```python
from build123d import *

# Parameters (mm, degrees)
F0_W     = 19.05
F0_H     = 3.175
F1_DEPTH = 9.525
F2_W     = 50.8
F2_H     = 6.35
F3_DEPTH = 12.7
F5_DEPTH = 273.051
F7_DEPTH = 19.05
F8_DEPTH = 19.05


with BuildPart() as f1:
    # F0 (on Top) → F1 (new body, symmetric)
    with BuildSketch(Plane.XY):
        Polygon((-127, 0), (127, 0), (127, 9.525), (-127, 9.525), (-127, 3.175), align=None)
        Polygon((-127, -3.175), (-127, -9.525), (127, -9.525), (127, 0), (-127, 0), align=None)
        with Locations((-136.525, 1.5875)):
            Rectangle(F0_W, F0_H)
        with Locations((-136.525, -1.5875)):
            Rectangle(F0_W, F0_H)
    extrude(amount=F1_DEPTH, both=True)

    # F2 (on Top) → F3 (cut, symmetric)
    with BuildSketch(Plane.XY):
        with Locations((101.6, 6.35)):
            Rectangle(F2_W, F2_H)
        with Locations((101.6, -6.35)):
            Rectangle(F2_W, F2_H)
    extrude(amount=F3_DEPTH, both=True, mode=Mode.SUBTRACT)

    # F4 (on face) → F5 (cut, through all)
    with BuildSketch(Plane.YZ.offset(127)):
        with BuildLine():
            ThreePointArc((-9.525, 0), (-7.77713, 5.499261), (-3.175, 8.980256))
            Line((-3.175, 8.980256), (-3.175, 9.525))
            Line((-3.175, 9.525), (-9.525, 9.525))
            Line((-9.525, 9.525), (-9.525, 0))
        make_face()
        with BuildLine():
            Line((-3.175, -9.525), (-3.175, -8.980256))
            ThreePointArc((-3.175, -8.980256), (-7.77713, -5.499261), (-9.525, 0))
            Line((-9.525, 0), (-9.525, -9.525))
            Line((-9.525, -9.525), (-3.175, -9.525))
        make_face()
        with BuildLine():
            Line((9.525, -9.525), (9.525, 0))
            ThreePointArc((9.525, 0), (7.77713, -5.499261), (3.175, -8.980256))
            Line((3.175, -8.980256), (3.175, -9.525))
            Line((3.175, -9.525), (9.525, -9.525))
        make_face()
        with BuildLine():
            ThreePointArc((3.175, 8.980256), (7.77713, 5.499261), (9.525, 0))
            Line((9.525, 0), (9.525, 9.525))
            Line((9.525, 9.525), (3.175, 9.525))
            Line((3.175, 9.525), (3.175, 8.980256))
        make_face()
        with BuildLine():
            ThreePointArc((0, 9.525), (1.610696, 9.387826), (3.175, 8.980256))
            Line((3.175, 8.980256), (3.175, 9.525))
            Line((3.175, 9.525), (0, 9.525))
        make_face()
        with BuildLine():
            ThreePointArc((-3.175, 8.980256), (-1.610696, 9.387826), (0, 9.525))
            Line((0, 9.525), (-3.175, 9.525))
            Line((-3.175, 9.525), (-3.175, 8.980256))
        make_face()
        with BuildLine():
            Line((-3.175, -9.525), (0, -9.525))
            ThreePointArc((0, -9.525), (-1.610696, -9.387826), (-3.175, -8.980256))
            Line((-3.175, -8.980256), (-3.175, -9.525))
        make_face()
        with BuildLine():
            Line((3.175, -9.525), (3.175, -8.980256))
            ThreePointArc((3.175, -8.980256), (1.610696, -9.387826), (0, -9.525))
            Line((0, -9.525), (3.175, -9.525))
        make_face()
    extrude(amount=-F5_DEPTH, mode=Mode.SUBTRACT)

    # F6 (on face) → F7 (cut)
    with BuildSketch(Plane(origin=(-146.05, 0, 0), x_dir=(0, -1, 0), z_dir=(-1, 0, 0))):
        with BuildLine():
            ThreePointArc((-3.175, 0), (0, 3.175), (3.175, 0))
            Line((3.175, 0), (3.175, 8.980256))
            ThreePointArc((3.175, 8.980256), (1.610696, 9.387826), (0, 9.525))
            ThreePointArc((0, 9.525), (-1.610696, 9.387826), (-3.175, 8.980256))
            Line((-3.175, 8.980256), (-3.175, 0))
        make_face()
    extrude(amount=-F7_DEPTH, mode=Mode.SUBTRACT)

    # F6 (on face) → F8 (cut)
    with BuildSketch(Plane(origin=(-146.05, 0, 0), x_dir=(0, -1, 0), z_dir=(-1, 0, 0))):
        with BuildLine():
            Line((3.175, -8.980256), (3.175, 0))
            ThreePointArc((3.175, 0), (0, -3.175), (-3.175, 0))
            Line((-3.175, 0), (-3.175, -8.980256))
            ThreePointArc((-3.175, -8.980256), (-1.610696, -9.387826), (0, -9.525))
            ThreePointArc((0, -9.525), (1.610696, -9.387826), (3.175, -8.980256))
        make_face()
    extrude(amount=-F8_DEPTH, mode=Mode.SUBTRACT)


solid = f1.part
```
Read the model definition and answer for the solid it produces. Units are mm, in the model's axes. A direction names the side the tool comes from. Coordinates: 2 decimals unless noted, no trailing zeros. Order: outer loops, then holes, each group sorted by start corner. A loop starts at its lowest first (then second) coordinate and runs counter-clockwise, first axis right, second up. Notation, with made-up numbers: (-30.75, -30.5) - (-19.75, -30.5) arc R14 ccw to (-19.75, -26.5) - close; hole circle Ø11 at (-34.75, 31). An arc over 180 degrees is marked (long way). Answer as a JSON object with one key per item and string values. Group by question number.
Item 1: Section C-C (y = 5.75) is taken. Give the vertices of the cut face in (x, z), plus the area to 3 significant figures.
Item 2: Section A-A (x = -44) is taken. Give the vertices of the cut face in (y, z) (3 decimals), plus the area to 3 significant figures.
Item 3: Section D-D (y = -7.25) is taken. Give the vertices of the cut face in (x, z), plus the area to 3 significant figures.
Item 4: A tool of negligible diameter and unlimited length cuts with its end or side. For faces 1 (the face through (76.2, 6, 0)), 2 (the face through (76.2, -6, 0)), 3 (the face through (-127, -4, 0)), 4 (the face through (-146.05, 0, 0)), 5 (the face through (127, 0, 0)), from which of +Z, -Z, +X, -X, +Y, -Y can it reach the whole face along a straight path? Write none if from no direction.
Item 5: Flat-ended cylindrical pins translate along their axes: P1, Ø1.5, axis at x = -1, y = -1, coming from the +Z side; P2, Ø1, axis at y = 7.5, z = -0.5, coming from the -X side; P3, Ø3, axis at y = 5, z = -2, coming from the +X side; P4, Ø5, axis at x = -39, z = 2.5, coming from the +Y side (3 decimals). Find the tip coordinate at first contact, or state that the pin passes through.
Item 6: Section B-B (z = -6.25) is taken. Give the vertices of the cut face in (x, y) (3 decimals), plus the area to 3 significant figures.
Item 7: Consider probe 1 along X at (y, z) = (-1, 4.5); probe 2 along X at (y, z) = (3.75, -1.75); probe 3 along Y at (x, z) = (116.5, 6) (3 decimals). Determine where each line is inside the solid, lowest interval first. Write a range as from..to.
Results are:
{
 "1": {"outline": "(-127, -7.59) - (76.2, -7.59) - (76.2, 7.59) - (-127, 7.59) - close", "area": "3,090 mm^2"},
 "2": {"outline": "(-3.175, -8.98) arc R9.525 ccw to (0, -9.525) arc R9.525 ccw to (3.175, -8.98) arc R9.525 ccw to (3.175, 8.98) arc R9.525 ccw to (0, 9.525) arc R9.525 ccw to (-3.175, 8.98) arc R9.525 ccw to start", "area": "285 mm^2"},
 "3": {"outline": "(-127, -6.18) - (76.2, -6.18) - (76.2, 6.18) - (-127, 6.18) - close", "area": "2,510 mm^2"},
 "4": {"face 1": "+Z, -Z, +X, +Y", "face 2": "+Z, -Z, +X, -Y", "face 3": "-X", "face 4": "+Z, -Z, -X, +Y, -Y", "face 5": "+Z, -Z, +X, +Y, -Y"},
 "5": {"P1": "stops at z = 9.52", "P2": "stops at x = -127", "P3": "stops at x = 76.2", "P4": "stops at y = 9.525"},
 "6": {"outline": "(-127, -7.188) - (76.2, -7.188) - (76.2, -3.175) - (127, -3.175) - (127, 3.175) - (76.2, 3.175) - (76.2, 7.188) - (-127, 7.188) - close", "area": "3,240 mm^2"},
 "7": {"probe 1": "x = -127..127", "probe 2": "x = -127..76.2", "probe 3": "y = -3.175..3.175"}
}
